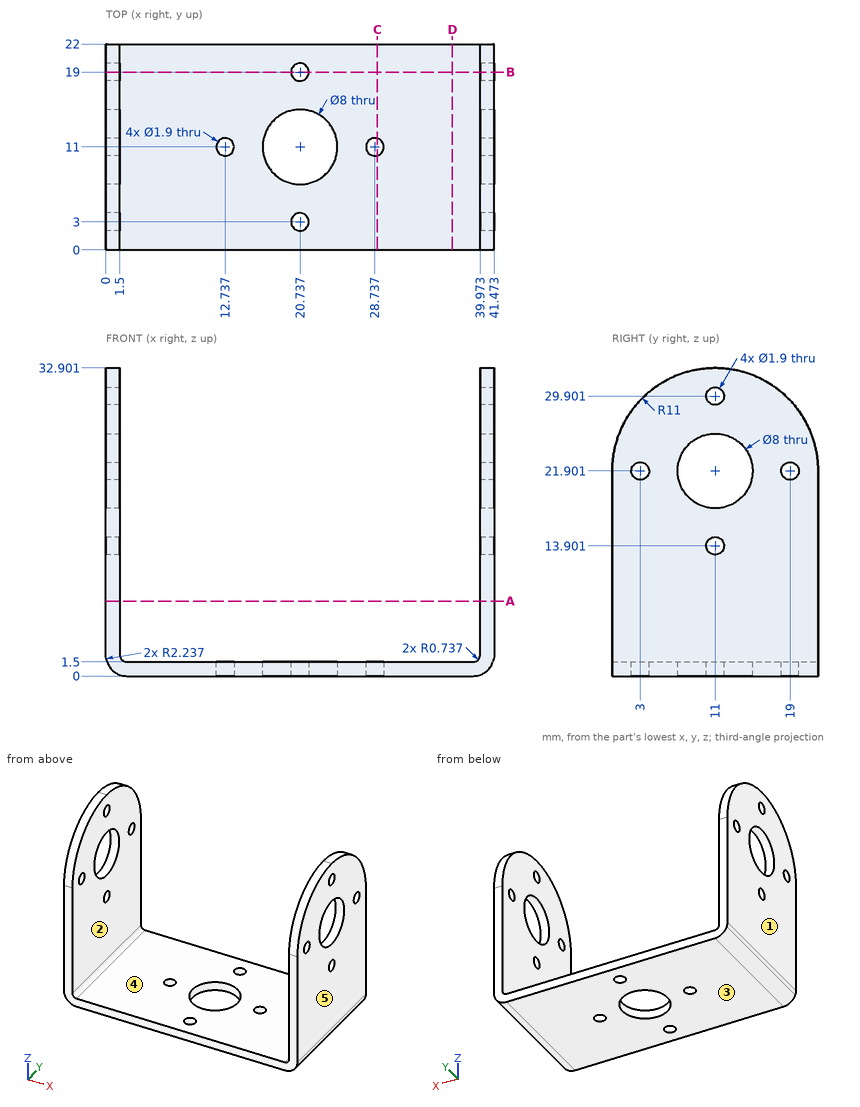
Geometry: see drawing. Coordinates: mm, zero at the bounding-box minimum. A direction names the side the tool comes from. Give positions to 0.01 mm unless a question says otherwise; leave off trailing zeros. Order: outer loops, then holes, each group sorted by start corner. A loop starts at its lowest first (then second) coordinate and runs counter-clockwise, first axis right, second up. Notation, with made-up numbers: (64.5, 79.5) - (75.5, 79.5) arc R20 ccw to (75.5, 84.5) - close; hole circle Ø6 at (-24, 52.25). An arc over 180 degrees is marked (long way). One line per item, written item: value.
1. Cut plane C-C, the plane x = 29. Output: boundary loops of the cut face in (y, z).
Determined:
outline: (0, 0) - (10.09, 0) - (10.09, 1.5) - (0, 1.5) - close; (11.91, 0) - (22, 0) - (22, 1.5) - (11.91, 1.5) - close
2. Cut plane B-B, the plane y = 19. Output: boundary loops of the cut face in (x, z) (1 decimal).
Determined:
outline: (0, 2.2) arc R2.2 ccw to (2.2, 0) - (19.8, 0) - (19.8, 1.5) - (2.2, 1.5) arc R0.7 cw to (1.5, 2.2) - (1.5, 21) - (0, 21) - close; (0, 22.9) - (1.5, 22.9) - (1.5, 29.5) - (0, 29.5) - close; (21.7, 0) - (39.2, 0) arc R2.2 ccw to (41.5, 2.2) - (41.5, 21) - (40, 21) - (40, 2.2) arc R0.7 cw to (39.2, 1.5) - (21.7, 1.5) - close; (40, 22.9) - (41.5, 22.9) - (41.5, 29.5) - (40, 29.5) - close
3. Line query: probe 1 along X at (y, z) = (13.5, 10); probe 2 along Z at (x, y) = (35.5, 2.75); probe 3 along X at (y, z) = (18.5, 2) (1 decimal). Output: solid intervals per line, ascending.
Determined:
probe 1: 0 to 1.5, 39.97 to 41.47
probe 2: 0 to 1.5
probe 3: 0 to 1.5, 39.9 to 41.5
4. Draft query along X for the marked faces 1, 2 and 3. Return one class per face: released by +X, released by -X, zero draft, split by the parting line, or undercut.
Determined:
face 1: released by -X
face 2: undercut
face 3: zero draft
5. Reachability of the marked faces 4 and 5 from +Z, -Z, +X, -X, +Y, -Y: full face, straight path, thin tool, end or side. Return the list, or none.
Determined:
face 4: +Z, +Y, -Y
face 5: +Z, -Z, +X, +Y, -Y
6. Pin query (flat end, axial travel): pin 1 Ø2.5 at (x, y) = (28.74, 11) entering from +Z; pin 2 Ø3 at (y, z) = (3, 21.9) entering from +X. Return the tip coordinate at first contact, or that it passes through.
Determined:
pin 1: z = 1.5
pin 2: x = 41.47
7. Cut plane A-A, the plane z = 8. Output: boundary loops of the cut face in (x, y).
Determined:
outline: (0, 0) - (1.5, 0) - (1.5, 22) - (0, 22) - close; (39.97, 0) - (41.47, 0) - (41.47, 22) - (39.97, 22) - close
8. Cut plane D-D, the plane x = 37. Output: boundary loops of the cut face in (y, z), and give its area (3 significant figures).
Determined:
outline: (0, 0) - (22, 0) - (22, 1.5) - (0, 1.5) - close
area: 33.0 mm2
